The model under review builds one solid part; all positions refer to its coordinate system, in mm. Face numbers are marked on the shaded views. A direction names the side the tool comes from. Give positions to 0.01 mm unless a question says otherwise; leave off trailing zeros. Order: outer loops, then holes, each group sorted by start corner. A loop starts at its lowest first (then second) coordinate and runs counter-clockwise, first axis right, second up.
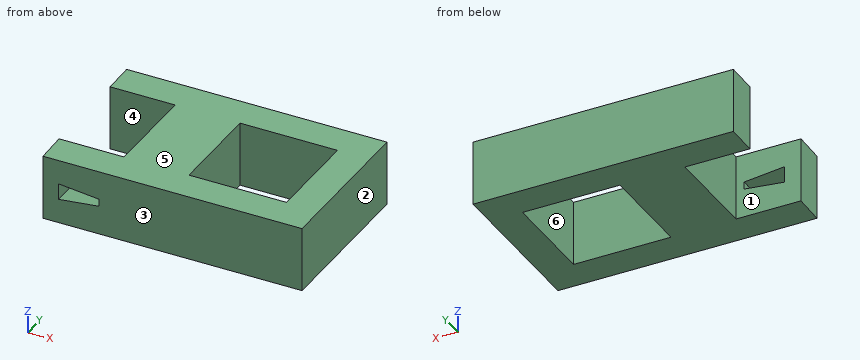
Autodesk Fusion 360 part; units mm, degrees
sketch "Sketch1" plane through (0, 0, 0) normal (0, 0, 1) x (1, 0, 0)
  line L0 (29.848, 60) -> (110, 60)
  line L1 (110, 60) -> (110, 10.0866)
  line L2 (110, 10.0866) -> (30.2597, 10.0866)
  line L3 (100, 50) -> (70, 50)
  line L4 (70, 50) -> (70, 20)
  line L5 (70, 20) -> (100, 20)
  line L6 (100, 20) -> (100, 50)
  line L7 (30, 50) -> (50, 50)
  line L8 (50, 50) -> (50, 20)
  line L9 (50, 20) -> (30, 20)
  line L10 (29.848, 60) -> (30, 50)
  line L11 (30, 20) -> (30.2597, 10.0866)
extrude "Extrude1" add sketch "Sketch1" along normal blind 20
sketch "Sketch2" plane through (0, 10.0866, 0) normal (0, -1, 0) x (1, 0, 0)
  line L0 (30.2597, 0) -> (110, 0)
  line L1 (110, 0) -> (110, 20)
  line L2 (110, 20) -> (30.2597, 20)
  line L3 (30.2597, 20) -> (30.2597, 0)
  line L4 (47.5008, 8.9134) -> (47.5008, 11.176)
  line L5 (35, 12.5) -> (35, 7.5)
  line L6 (35, 7.5) -> (47.5008, 8.9134)
  line L7 (35, 12.5) -> (47.5008, 11.176)
  line L8 (47.6079, 8.9255) -> (47.5008, 9.8724)
extrude "Extrude2" cut sketch "Sketch2" against normal blind 11 contours L4 L5 L6 L7
Item 1: Draft analysis for pull direction Y (two halves, no side actions). For the marked faces 1, 2 and 3, state which applies: released by +Y, released by -Y, zero draft, split by the parting line, or undercut.
Values found:
face 1: undercut
face 2: zero draft
face 3: released by -Y
Item 2: Take a section at B-B (z = 5). Give the boundary of the cut face in (x, y).
Values found:
outline: (29.85, 60) - (30, 50) - (50, 50) - (50, 20) - (30, 20) - (30.26, 10.09) - (110, 10.09) - (110, 60) - close; hole (70, 20) - (100, 20) - (100, 50) - (70, 50) - close
Item 3: For line 1 (Y direction, x = 40.5, z = 5.5); line 2 (X direction, y = 48.5, z = 14.75); line 3 (Z direction, x = 38.5, y = 14), list the stretches that pass through material, from the lowest coordinate up.
Values found:
line 1: y = 10.09 to 20, 50 to 60
line 2: x = 50 to 70, 100 to 110
line 3: z = 0 to 7.9, 12.13 to 20
Item 4: Take a section at C-C (x = 82.5). Give the boundary of the cut face in (y, z), and give its area (3 significant figures).
Values found:
outline: (10.09, 0) - (20, 0) - (20, 20) - (10.09, 20) - close; (50, 0) - (60, 0) - (60, 20) - (50, 20) - close
area: 398 mm2
Item 5: Clearance check with flat-ended pins moving along their axes: pin 1 Ø10 at (x, y) = (75, 16) entering from -Z; pin 2 Ø1.5 at (y, z) = (52, 10.5) entering from -X; pin 3 Ø0.7 at (y, z) = (17.5, 10) entering from -X. State where each tip first meets the part, or that it passes through.
Values found:
pin 1: stops at z = 0
pin 2: stops at x = 29.96
pin 3: stops at x = 30.06
Item 6: Take a section at A-A (y = 37.5). Give the boundary of the cut face in (x, z).
Values found:
outline: (50, 0) - (70, 0) - (70, 20) - (50, 20) - close; (100, 0) - (110, 0) - (110, 20) - (100, 20) - close
Item 7: Take a section at D-D (x = 45.5). Give the boundary of the cut face in (y, z).
Values found:
outline: (10.09, 0) - (20, 0) - (20, 8.69) - (10.09, 8.69) - close; (10.09, 11.39) - (20, 11.39) - (20, 20) - (10.09, 20) - close; (50, 0) - (60, 0) - (60, 20) - (50, 20) - close
Item 8: For the marked faces 4, 5 and 6, list the 3-axis set-ups (+Z, -Z, +X, -X, +Y, -Y) from which the entire face can be reached by the end or side of a thin tool; tool diameter is ignored.
Values found:
face 4: +Z, -Z, -X
face 5: +Z, +X, -X, +Y, -Y
face 6: +Z, -Z
